from build123d import *

# Parameters (mm, degrees)
SKETCH1_W           = 30
SKETCH1_H           = 22
SKETCH1_H_2         = 32
SKETCH1_R           = 2.5
BOSS_EXTRUDE1_DEPTH = 20


with BuildPart() as part:
    # Sketch1 → Boss-Extrude1 (new body)
    # profile 1 of 2: a face of its own
    with BuildSketch(Plane(origin=(0, 0, 0), x_dir=(1, 0, 0), z_dir=(0, 1, 0))):
        with Locations((0, 3.5)):
            Rectangle(SKETCH1_W, SKETCH1_H)
        with BuildLine():
            ThreePointArc((-7.5, -2.5), (-10, -5), (-12.5, -2.5))
            Line((-12.5, -2.5), (-12.5, 0))
            Line((-12.5, 0), (-12.5, 2.5))
            ThreePointArc((-12.5, 2.5), (-10, 5), (-7.5, 2.5))
            Line((-7.5, 2.5), (-7.5, 0))
            Line((-7.5, 0), (-7.5, -2.5))
        make_face(mode=Mode.SUBTRACT)
        with BuildLine():
            ThreePointArc((12.5, -2.5), (10, -5), (7.5, -2.5))
            Line((7.5, -2.5), (7.5, 0))
            Line((7.5, 0), (7.5, 2.5))
            ThreePointArc((7.5, 2.5), (10, 5), (12.5, 2.5))
            Line((12.5, 2.5), (12.5, 0))
            Line((12.5, 0), (12.5, -2.5))
        make_face(mode=Mode.SUBTRACT)
    # profile 2 of 2: a face of its own
    with BuildSketch(Plane(origin=(0, 0, 0), x_dir=(1, 0, 0), z_dir=(0, 1, 0))):
        with Locations((0, 3.5)):
            Rectangle(SKETCH1_W, SKETCH1_H_2)
        with Locations(Location((10, 0, 0), (0, 0, 270))):
            Circle(SKETCH1_R, mode=Mode.SUBTRACT)
        with Locations(Location((-10, 0, 0), (0, 0, 270))):
            Circle(SKETCH1_R, mode=Mode.SUBTRACT)
    extrude(amount=BOSS_EXTRUDE1_DEPTH)


solid = part.part
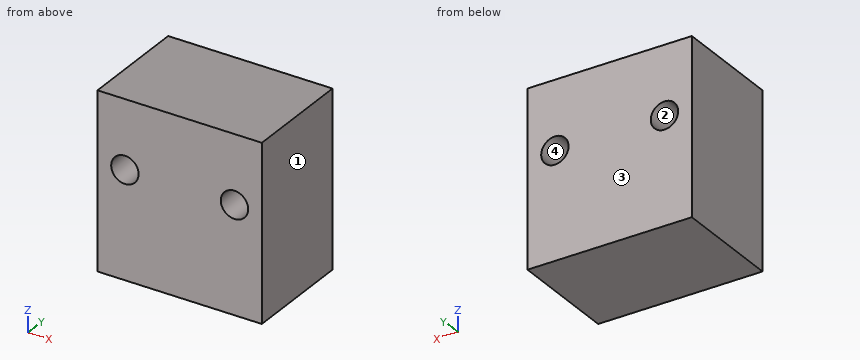
The model under review builds one solid part; all positions refer to its coordinate system, in mm. Face numbers are marked on the shaded views. Give positions to 0.01 mm unless a question says otherwise; leave off trailing zeros. Write each loop counter-clockwise with the first axis right and the second up, starting at its lowest first coordinate (ties: lowest second). Pieces come first, ordered by that corner, then holes.
1. Draft analysis for pull direction X (two halves, no side actions). For the marked faces 1, 2, 3 and 4, state which applies: +X half, -X half, draft (parallel to the pull), parting line (faces both ways), or undercut.
2. For P1, Ø4.5, axis at x = 10, z = 0, coming from the -Y side, flat-tipped, find the tip position at first contact; note if it passes through.
3. Add section A-A, the plane z = 0. Write out the cut boundary in (x, y).
4. Wall thickness on L1, parallel to X at y = 14.5, z = 0; L2, parallel to Z at x = -10, y = 9.75; L3, parallel to X at y = 4.5, z = 1: over which ranges is each line inside the solid? List them lowest first.
5. Add section D-D, the plane x = 11. Write out the cut boundary in (y, z).
6. Add section C-C, the plane y = 2.5. Write out the cut boundary in (x, z).
7. Add section B-B, the plane x = -10. Write out the cut boundary in (y, z).
Worked answers:
1. face 1: +X half
1. face 2: undercut
1. face 3: draft
1. face 4: undercut
2. P1: passes through
3. outline: (-15, 0) - (-12.5, 0) - (-12.5, 20) - (-15, 20) - close; (-7.5, 0) - (7.5, 0) - (7.5, 20) - (-7.5, 20) - close; (12.5, 0) - (15, 0) - (15, 20) - (12.5, 20) - close
4. L1: x = -15 to -12.5, -7.5 to 7.5, 12.5 to 15
4. L2: z = -19.5 to -2.5, 2.5 to 12.5
4. L3: x = -15 to -12.29, -7.71 to 7.71, 12.29 to 15
5. outline: (0, -19.5) - (20, -19.5) - (20, -2.29) - (0, -2.29) - close; (0, 2.29) - (20, 2.29) - (20, 12.5) - (0, 12.5) - close
6. outline: (-15, -19.5) - (15, -19.5) - (15, 12.5) - (-15, 12.5) - close; hole circle Ø5 at (-10, 0); hole circle Ø5 at (10, 0)
7. outline: (0, -19.5) - (20, -19.5) - (20, -2.5) - (0, -2.5) - close; (0, 2.5) - (20, 2.5) - (20, 12.5) - (0, 12.5) - close
